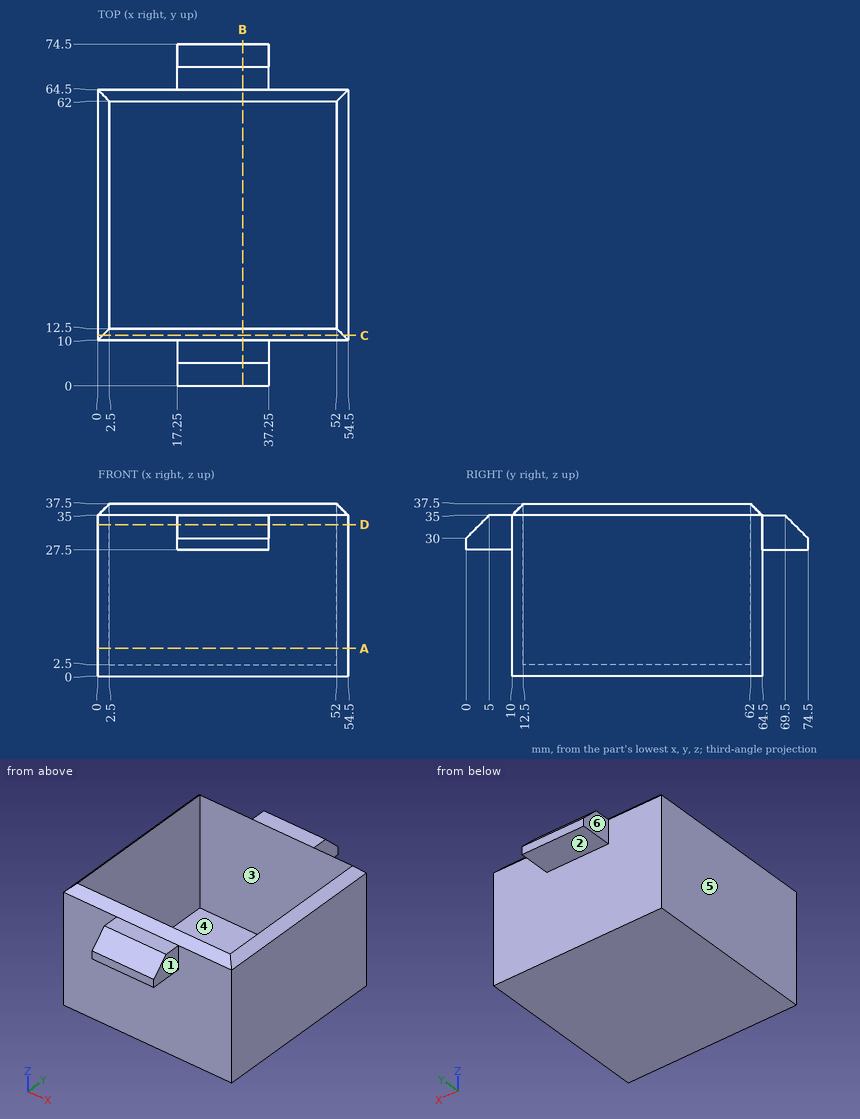
Drawing for the job (mm, zero at the part's lowest x, y, z). A direction names the side the tool comes from. Coordinates: 2 decimals unless noted, no trailing zeros. Order: outer loops, then holes, each group sorted by start corner. A loop starts at its lowest first (then second) coordinate and runs counter-clockwise, first axis right, second up.
Item 1: Band-saw the part on A-A on z = 6. List the corners of the cut face in (x, y).
Check sheet entries:
outline: (0, 10) - (54.5, 10) - (54.5, 64.5) - (0, 64.5) - close; hole (2.5, 12.5) - (52, 12.5) - (52, 62) - (2.5, 62) - close
Item 2: Drill centre lines: L1, parallel to X at y = 56.5, z = 34.5; L2, parallel to Y at x = 11.5, z = 20; L3, parallel to Y at x = 34, z = 30. Where is each one in solid material? Low to high.
Check sheet entries:
L1: x = 0 to 2.5, 52 to 54.5
L2: y = 10 to 12.5, 62 to 64.5
L3: y = 0 to 12.5, 62 to 74.5
Item 3: Two-plate mould, pull along X, no slides. Class the marked faces 1, 2 and 3: +X half, -X half, draft (parallel to the pull), parting line (faces both ways), or undercut.
Check sheet entries:
face 1: +X half
face 2: draft
face 3: undercut
Item 4: Pin check, flat tips, straight feed: pin 1 Ø2 at (x, z) = (43.5, 19) entering from +Y; pin 2 Ø4 at (y, z) = (68, 31.5) entering from +X; pin 3 Ø12 at (x, z) = (42, 12) entering from -Y. Stop position of each tip, or through.
Check sheet entries:
pin 1: stops at y = 64.5
pin 2: stops at x = 37.25
pin 3: stops at y = 10
Item 5: Band-saw the part on B-B on x = 31.5. List the corners of the cut face in (y, z).
Check sheet entries:
outline: (0, 27.5) - (10, 27.5) - (10, 0) - (64.5, 0) - (64.5, 27.5) - (74.5, 27.5) - (74.5, 30) - (69.5, 35) - (64.5, 35) - (62, 37.5) - (62, 2.5) - (12.5, 2.5) - (12.5, 37.5) - (10, 35) - (5, 35) - (0, 30) - close
Item 6: 3-axis set-ups, long thin cutter, end or side, ignore diameter. For the marked faces 4, 5 and 6: which of +Z, -Z, +X, -X, +Y, -Y reach the whole face in a straight line?
Check sheet entries:
face 4: +Z
face 5: +Z, -Z, -X, +Y, -Y
face 6: +Z, -Z, -X, +Y
Item 7: Band-saw the part on C-C on y = 11. List the corners of the cut face in (x, z).
Check sheet entries:
outline: (0, 0) - (54.5, 0) - (54.5, 35) - (53.5, 36) - (1, 36) - (0, 35) - close
Item 8: Band-saw the part on D-D on z = 33. List the corners of the cut face in (x, y).
Check sheet entries:
outline: (0, 10) - (17.25, 10) - (17.25, 3) - (37.25, 3) - (37.25, 10) - (54.5, 10) - (54.5, 64.5) - (37.25, 64.5) - (37.25, 71.5) - (17.25, 71.5) - (17.25, 64.5) - (0, 64.5) - close; hole (2.5, 12.5) - (52, 12.5) - (52, 62) - (2.5, 62) - close
